```python
from build123d import *

# Parameters (mm, degrees)
SKETCH1_R            = 1.450000006
SKETCH1_R_2          = 1.449941928
SKETCH1_W            = 6.2
SKETCH1_H            = 3.4
SKETCH1_R_3          = 1.450000003
SKETCH1_R_4          = 40
SKETCH1_R_5          = 1.45
BOSS_EXTRUDE11_DEPTH = 5.85


with BuildPart() as part:
    # Sketch1 → Boss-Extrude11 (new body)
    with BuildSketch(Plane.XY):
        with BuildLine():
            ThreePointArc((639.724883257, 499.569822456), (638.966034957, 499.676986361), (638.266537412, 499.990096614))
            Line((638.266537412, 499.990096614), (588.077856055, 531.537433899))
            ThreePointArc((588.077856055, 531.537433899), (583.344226303, 531.18640109), (582.27874868, 526.560903053))
            Line((582.27874868, 526.560903053), (605.213170633, 473.617916038))
            Line((605.213170633, 473.617916038), (548.836184659, 455.29378772))
            ThreePointArc((548.836184659, 455.29378772), (546.073009962, 451.434339541), (548.941914767, 447.652823988))
            Line((548.941914767, 447.652823988), (554.763084266, 445.937340724))
            Line((554.763084266, 445.937340724), (596.245460931, 433.712593969))
            Line((596.245460931, 433.712593969), (599.290728508, 432.815161663))
            Line((599.290728508, 432.815161663), (604.285764635, 431.343137719))
            Line((604.285764635, 431.343137719), (582.236160138, 376.31629729))
            ThreePointArc((582.236160138, 376.31629729), (583.429213887, 371.72205117), (588.170744102, 371.502128745))
            Line((588.170744102, 371.502128745), (592.100192099, 374.12650821))
            Line((592.100192099, 374.12650821), (603.596221534, 381.804417066))
            Line((603.596221534, 381.804417066), (636.150805744, 403.546804888))
            ThreePointArc((636.150805744, 403.546804888), (636.852224463, 403.859925316), (637.612849666, 403.967079047))
            Line((637.612849666, 403.967079047), (662.711272535, 403.967079047))
            ThreePointArc((662.711272535, 403.967079047), (663.470120836, 403.859915142), (664.16961838, 403.546804888))
            Line((664.16961838, 403.546804888), (712.149680023, 371.502128745))
            ThreePointArc((712.149680023, 371.502128745), (716.891210238, 371.72205117), (718.084263987, 376.31629729))
            Line((718.084263987, 376.31629729), (696.03465949, 431.343137719))
            Line((696.03465949, 431.343137719), (751.378509358, 447.652823988))
            ThreePointArc((751.378509358, 447.652823988), (754.247414163, 451.434339541), (751.484239466, 455.29378772))
            Line((751.484239466, 455.29378772), (745.965056767, 457.087679505))
            Line((745.965056767, 457.087679505), (702.479915956, 471.221590468))
            Line((702.479915956, 471.221590468), (695.107253492, 473.617916038))
            Line((695.107253492, 473.617916038), (701.597430802, 488.600171695))
            Line((701.597430802, 488.600171695), (702.867715773, 491.532562182))
            Line((702.867715773, 491.532562182), (714.311493474, 517.949961123))
            Line((714.311493474, 517.949961123), (718.041675445, 526.560903053))
            ThreePointArc((718.041675445, 526.560903053), (716.976197822, 531.18640109), (712.24256807, 531.537433899))
            Line((712.24256807, 531.537433899), (662.053886713, 499.990096614))
            ThreePointArc((662.053886713, 499.990096614), (661.354389168, 499.676986361), (660.595540868, 499.569822456))
            Line((660.595540868, 499.569822456), (639.724883257, 499.569822456))
        make_face()
        with Locations((585.949161838, 374.828473923)):
            Circle(SKETCH1_R, mode=Mode.SUBTRACT)
        with BuildLine():
            Line((624.68020842, 401.06117225), (591.294683214, 379.029224839))
            ThreePointArc((591.294683214, 379.029224839), (589.396544209, 379.138356483), (588.959649961, 380.988752337))
            Line((588.959649961, 380.988752337), (590.118736999, 383.663703413))
            Line((590.118736999, 383.663703413), (604.863272518, 417.69126982))
            ThreePointArc((604.863272518, 417.69126982), (605.13587571, 417.91953965), (605.481867106, 417.837627687))
            Line((605.481867106, 417.837627687), (624.718077603, 401.725200151))
            ThreePointArc((624.718077603, 401.725200151), (624.865817134, 401.383680858), (624.68020842, 401.06117225))
        make_face(mode=Mode.SUBTRACT)
        with Locations((624.115265697, 417.388768355)):
            Circle(SKETCH1_R_2, mode=Mode.SUBTRACT)
        with Locations((610.19862014, 424.360721889)):
            Rectangle(SKETCH1_W, SKETCH1_H, mode=Mode.SUBTRACT)
        with Locations((610.19862014, 432.360721889)):
            Circle(SKETCH1_R_3, mode=Mode.SUBTRACT)
        with Locations((650.160212062, 451.489683338)):
            Circle(SKETCH1_R_4, mode=Mode.SUBTRACT)
        with BuildLine():
            ThreePointArc((694.750680645, 417.792560251), (695.112666193, 417.878751085), (695.398044556, 417.639959152))
            Line((695.398044556, 417.639959152), (709.259881072, 385.64059016))
            Line((709.259881072, 385.64059016), (711.297941568, 380.935827572))
            ThreePointArc((711.297941568, 380.935827572), (710.860859499, 379.085476074), (708.962709426, 378.9765371))
            Line((708.962709426, 378.9765371), (675.579420729, 401.011873172))
            ThreePointArc((675.579420729, 401.011873172), (675.401955879, 401.319973549), (675.54270419, 401.646484695))
            Line((675.54270419, 401.646484695), (694.750680645, 417.792560251))
        make_face(mode=Mode.SUBTRACT)
        with Locations((714.371262287, 374.828473923)):
            Circle(SKETCH1_R, mode=Mode.SUBTRACT)
        with Locations((675.215266265, 417.413768355)):
            Circle(SKETCH1_R_2, mode=Mode.SUBTRACT)
        with Locations((690.19862014, 424.360721889)):
            Rectangle(SKETCH1_W, SKETCH1_H, mode=Mode.SUBTRACT)
        with Locations((690.19862014, 432.360721889)):
            Circle(SKETCH1_R_3, mode=Mode.SUBTRACT)
        with BuildLine():
            Line((704.657868853, 438.89520987), (704.635906667, 463.98787081))
            ThreePointArc((704.635906667, 463.98787081), (704.802560484, 464.320570227), (705.168923392, 464.38569024))
            Line((705.168923392, 464.38569024), (743.506176223, 452.972756989))
            ThreePointArc((743.506176223, 452.972756989), (744.642676768, 451.448549682), (743.506021515, 449.924457744))
            Line((743.506021515, 449.924457744), (705.167610421, 438.515415947))
            ThreePointArc((705.167610421, 438.515415947), (704.817519632, 438.577513089), (704.657868853, 438.89520987))
        make_face(mode=Mode.SUBTRACT)
        with Locations((750.247797049, 451.489683338)):
            Circle(SKETCH1_R, mode=Mode.SUBTRACT)
        with Locations((550.072627076, 451.489683338)):
            Circle(SKETCH1_R, mode=Mode.SUBTRACT)
        with BuildLine():
            Line((595.662555272, 464.084156807), (595.684517458, 438.991495867))
            ThreePointArc((595.684517458, 438.991495867), (595.517863641, 438.65879645), (595.151500732, 438.593676437))
            Line((595.151500732, 438.593676437), (556.814247902, 450.006609688))
            ThreePointArc((556.814247902, 450.006609688), (555.677747357, 451.530816994), (556.81440261, 453.054908933))
            Line((556.81440261, 453.054908933), (560.257551409, 454.079547864))
            Line((560.257551409, 454.079547864), (595.152813704, 464.46395073))
            ThreePointArc((595.152813704, 464.46395073), (595.502904493, 464.401853588), (595.662555272, 464.084156807))
        make_face(mode=Mode.SUBTRACT)
        with Locations((610.19862014, 471.710721889)):
            Circle(SKETCH1_R_3, mode=Mode.SUBTRACT)
        with Locations((610.19862014, 479.710721889)):
            Rectangle(SKETCH1_W, SKETCH1_H, mode=Mode.SUBTRACT)
        with Locations((624.115265697, 486.43876853)):
            Circle(SKETCH1_R_2, mode=Mode.SUBTRACT)
        with Locations((585.949161838, 528.150892754)):
            Circle(SKETCH1_R, mode=Mode.SUBTRACT)
        with BuildLine():
            Line((604.922379569, 485.339407525), (589.022482557, 522.043539105))
            ThreePointArc((589.022482557, 522.043539105), (589.459564626, 523.893890603), (591.357714699, 524.002829577))
            Line((591.357714699, 524.002829577), (596.297768126, 520.742044264))
            Line((596.297768126, 520.742044264), (624.741003396, 501.967493505))
            ThreePointArc((624.741003396, 501.967493505), (624.918468246, 501.659393128), (624.777719935, 501.332881982))
            Line((624.777719935, 501.332881982), (605.56974348, 485.186806426))
            ThreePointArc((605.56974348, 485.186806426), (605.207757932, 485.100615592), (604.922379569, 485.339407525))
        make_face(mode=Mode.SUBTRACT)
        with Locations((636.087236238, 493.259844204)):
            Circle(SKETCH1_R_5, mode=Mode.SUBTRACT)
        with Locations((650.160212062, 493.259844204)):
            Circle(SKETCH1_R_5, mode=Mode.SUBTRACT)
        with Locations((675.215266265, 486.46376853)):
            Circle(SKETCH1_R_2, mode=Mode.SUBTRACT)
        with Locations((690.19862014, 471.710721889)):
            Circle(SKETCH1_R_3, mode=Mode.SUBTRACT)
        with Locations((690.19862014, 479.710721889)):
            Rectangle(SKETCH1_W, SKETCH1_H, mode=Mode.SUBTRACT)
        with Locations((664.233187887, 493.259844204)):
            Circle(SKETCH1_R_5, mode=Mode.SUBTRACT)
        with BuildLine():
            ThreePointArc((709.025740911, 523.950141838), (710.923879916, 523.841010194), (711.360774164, 521.99061434))
            Line((711.360774164, 521.99061434), (710.94300028, 521.026472162))
            Line((710.94300028, 521.026472162), (697.668691106, 490.391906812))
            Line((697.668691106, 490.391906812), (695.457151607, 485.288096857))
            ThreePointArc((695.457151607, 485.288096857), (695.184548415, 485.059827027), (694.838557019, 485.14173899))
            Line((694.838557019, 485.14173899), (675.602346522, 501.254166526))
            ThreePointArc((675.602346522, 501.254166526), (675.454606991, 501.595685819), (675.640215705, 501.918194427))
            Line((675.640215705, 501.918194427), (709.025740911, 523.950141838))
        make_face(mode=Mode.SUBTRACT)
        with Locations((714.371262287, 528.150892754)):
            Circle(SKETCH1_R, mode=Mode.SUBTRACT)
    extrude(amount=BOSS_EXTRUDE11_DEPTH)


solid = part.part
```
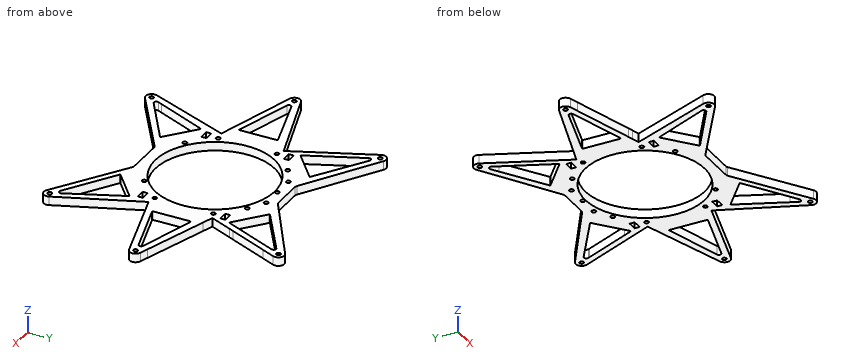
Work out the finished part from the listing and answer in its coordinate system (mm). Give positions to 0.01 mm unless a question says otherwise; leave off trailing zeros. Write each loop counter-clockwise with the first axis right and the second up, starting at its lowest first coordinate (ties: lowest second). Pieces come first, ordered by that corner, then holes. Notation, with made-up numbers: (34, 21) - (73, 21) arc R10 cw to (73, 30) - close; hole circle Ø1 at (-10, 46). An arc over 180 degrees is marked (long way). Use one line per item in the form item = value.
1. A cutting plane is placed at B-B (y = 497). Write down the section's boundary in (x, z).
Filled in:
outline = (595.08, 0) - (599.87, 0) - (599.87, 5.85) - (595.08, 5.85) - close; (619.62, 0) - (680.68, 0) - (680.68, 5.85) - (619.62, 5.85) - close; (700.53, 0) - (705.24, 0) - (705.24, 5.85) - (700.53, 5.85) - close
2. A cutting plane is placed at A-A (y = 388.5). Write down the section's boundary in (x, z).
Filled in:
outline = (587.12, 0) - (592.21, 0) - (592.21, 5.85) - (587.12, 5.85) - close; (605.65, 0) - (613.62, 0) - (613.62, 5.85) - (605.65, 5.85) - close; (686.7, 0) - (694.53, 0) - (694.53, 5.85) - (686.7, 5.85) - close; (708.02, 0) - (713.2, 0) - (713.2, 5.85) - (708.02, 5.85) - close
3. Each of these flat-tipped pins is pushed along its axis until it touches: pin 1 Ø1.7 at (y, z) = (424, 3.5) entering from +X; pin 2 Ø3 at (y, z) = (419.5, 1) entering from -X; pin 3 Ø3.5 at (y, z) = (479, 4) entering from -X. Where does it stop, or does it pass through?
Filled in:
pin_1 = 699.32
pin_2 = 598.94
pin_3 = 602.12
4. Consider L1, parallel to Y at x = 650, z = 1.35; L2, parallel to Y at x = 674.5, z = 2.6 (3 decimals); L3, parallel to Y at x = 695, z = 4.35. Determine where each line is inside the solid, lowest interval first.
Filled in:
L1 = 403.97 to 411.49, 491.49 to 491.82, 494.7 to 499.57
L2 = 396.647 to 416.153, 418.675 to 419.747, 483.232 to 485.203, 487.725 to 507.813
L3 = 382.96 to 388.19, 417.89 to 485.06, 514.69 to 520.7
5. A cutting plane is placed at C-C (z = 1.05). State how many separate pieces and enclosed holes the cut face has, and give its area (3 significant figures).
Filled in:
separate_pieces = 1
enclosed_holes = 28
area = 6,790 mm^2
